from build123d import *

# Parameters (mm, degrees)
SKETCH2_W           = 28.575
SKETCH2_H           = 22.225
BOSS_EXTRUDE1_DEPTH = 15.875
SKETCH5_W           = 19.05
SKETCH5_H           = 19.05
CUT_EXTRUDE3_DEPTH  = 12.7
SKETCH4_R           = 1.5875
CUT_EXTRUDE2_DEPTH  = 3.175
CUT_EXTRUDE1_DEPTH  = 23.225
SKETCH6_R           = 0.79375
CUT_EXTRUDE4_DEPTH  = 1.5875


with BuildPart() as part:
    # Sketch2 → Boss-Extrude1 (new body)
    with BuildSketch(Plane.XY):
        Rectangle(SKETCH2_W, SKETCH2_H)
    extrude(amount=BOSS_EXTRUDE1_DEPTH)

    # Sketch5 → Cut-Extrude3 (cut)
    with BuildSketch(Plane.XY.offset(15.875)):
        Rectangle(SKETCH5_W, SKETCH5_H)
    extrude(amount=-CUT_EXTRUDE3_DEPTH, mode=Mode.SUBTRACT)

    # Sketch4 → Cut-Extrude2 (cut)
    with BuildSketch(Plane.ZY.offset(14.2875)):
        with BuildLine():
            ThreePointArc((6.35, -5.55625), (3.175, -8.73125), (0, -5.55625))
            Line((0, -5.55625), (0, -11.1125))
            Line((0, -11.1125), (15.875, -11.1125))
            Line((15.875, -11.1125), (15.875, 11.1125))
            Line((15.875, 11.1125), (0, 11.1125))
            Line((0, 11.1125), (0, 5.55625))
            ThreePointArc((0, 5.55625), (3.175, 8.73125), (6.35, 5.55625))
            Line((6.35, 5.55625), (6.35, -5.55625))
        make_face()
        with Locations((3.175, 5.55625)):
            Circle(SKETCH4_R)
        with Locations((3.175, 0)):
            Circle(SKETCH4_R)
        with Locations((3.175, -5.55625)):
            Circle(SKETCH4_R)
    cut_extrude2 = extrude(amount=-CUT_EXTRUDE2_DEPTH, mode=Mode.SUBTRACT)

    # Mirror1: Cut-Extrude2 across plane
    add(cut_extrude2.mirror(Plane(origin=(0, 0, 0), x_dir=(0, 0, 1), z_dir=(1, 0, 0))), mode=Mode.SUBTRACT)

    # Sketch3 → Cut-Extrude1 (cut, through all)
    with BuildSketch(Plane(origin=(0, 11.1125, 0), x_dir=(1, 0, 0), z_dir=(0, 1, 0))):
        with BuildLine():
            Line((-7.9375, -6.35), (-9.525, -6.35))
            Line((-9.525, -6.35), (-9.525, -15.875))
            Line((-9.525, -15.875), (9.525, -15.875))
            Line((9.525, -15.875), (9.525, -6.35))
            Line((9.525, -6.35), (7.9375, -6.35))
            ThreePointArc((7.9375, -6.35), (0, -9.637820151), (-7.9375, -6.35))
        make_face()
    extrude(amount=-CUT_EXTRUDE1_DEPTH, mode=Mode.SUBTRACT)

    # Sketch6 → Cut-Extrude4 (cut)
    with BuildSketch(Plane.ZY.offset(11.1125)):
        with BuildLine():
            Line((15.875, -11.1125), (15.875, 0))
            add(Edge.make_bspline(
                [(6.35, -5.55625), (15.875, -2.778125), (15.875, 0)],
                knots=[0, 0, 0, 0.5, 0.5, 0.5], degree=2))
            Line((6.35, -5.55625), (6.35, -11.1125))
            Line((6.35, -11.1125), (15.875, -11.1125))
        make_face()
        with BuildLine():
            Line((6.35, 11.1125), (6.35, 5.55625))
            add(Edge.make_bspline(
                [(15.875, 0), (15.875, 2.778125), (6.35, 5.55625)],
                knots=[0.5, 0.5, 0.5, 1, 1, 1], degree=2))
            Line((15.875, 0), (15.875, 11.1125))
            Line((15.875, 11.1125), (6.35, 11.1125))
        make_face()
        with Locations((14.2875, 0)):
            Circle(SKETCH6_R)
    cut_extrude4 = extrude(amount=-CUT_EXTRUDE4_DEPTH, mode=Mode.SUBTRACT)

    # Mirror2: Cut-Extrude4 across plane
    add(cut_extrude4.mirror(Plane(origin=(0, 0, 0), x_dir=(0, 0, 1), z_dir=(1, 0, 0))), mode=Mode.SUBTRACT)


solid = part.part
Geometry check sheet. Reference: the model listing, model coordinates, mm. A direction names the side the tool comes from. Round coordinates to 2 decimals unless told otherwise and drop trailing zeros. Loops run counter-clockwise (first coordinate to the right, second up) from the corner with the lowest first, then second, coordinate; pieces in that order, holes last. Notation, with made-up numbers: (55, 74) - (113, 74) arc R18 cw to (113, 91) - close; hole circle Ø4 at (51, -29.75). An arc over 180 degrees is marked (long way). Answer as CSV lines item,"result".
(1) Cross-section at C-C, the plane x = 6. Enter the section's corners in (y, z) (1 decimal).
Output values:
outline,"(-11.1, 0) - (11.1, 0) - (11.1, 7.9) - (9.5, 7.9) - (9.5, 3.2) - (-9.5, 3.2) - (-9.5, 7.9) - (-11.1, 7.9) - close"
(2) Material ranges on line 1 along Y through (x, z) = (-2.75, 7) (1 decimal); line 2 along X through (y, z) = (-7.25, 4.5) (1 decimal), recorded low to high.
Output values:
line 1,"y = -11.1 to -9.5, 9.5 to 11.1"
line 2,"x = -14.3 to -9.5, 9.5 to 14.3"
(3) Cross-section at B-B, the plane z = 6. Enter the section's corners in (x, y) (1 decimal).
Output values:
outline,"(-14.3, -7) - (-11.1, -7) - (-11.1, -11.1) - (11.1, -11.1) - (11.1, -7) - (14.3, -7) - (14.3, 7) - (11.1, 7) - (11.1, 11.1) - (-11.1, 11.1) - (-11.1, 7) - (-14.3, 7) - close; hole (-9.5, -9.5) - (9.5, -9.5) - (9.5, 9.5) - (-9.5, 9.5) - close"
(4) Release check for a two-part mould opening along Z. For faces 1 (the face through (0, -11.112, 4)), 2 (the face through (-10, -9, 6.35)), 3 (the face through (10.33, 0.035, 13.495)) record: released by +Z, released by -Z, zero draft, split by the parting line, or undercut.
Output values:
face 1,"zero draft"
face 2,"released by +Z"
face 3,"undercut"
(5) Set-up check for faces 4 (the face through (-11.112, 0, 10)), 5 (the face through (0, 9.525, 6)), 6 (the face through (10, -9, 6.35)): record each of +Z, -Z, +X, -X, +Y, -Y from which the full face is reachable in a straight line by a thin tool's end or side.
Output values:
face 4,"+Z, -X, +Y, -Y"
face 5,"+Z"
face 6,"+Z, +X, -Y"
(6) Depth check by flat-ended pin: pin 1 Ø1.7 at (y, z) = (9, 2) entering from +X; pin 2 Ø1.6 at (y, z) = (-5.5, 3.5) entering from -X; pin 3 Ø2.5 at (y, z) = (0, 14.29) entering from +X; pin 4 Ø2 at (x, y) = (-2, -8) entering from +Z (3 decimals). Enter the tip coordinate at first touch or a pass-through.
Output values:
pin 1,"stops at x = 14.29"
pin 2,"stops at x = -11.11"
pin 3,"stops at x = 11.11"
pin 4,"stops at z = 3.175"
